Autodesk Inventor part; units mm, degrees
ref_plane "YZ Plane" through (0, 0, 0) normal (1, 0, 0) x (0, 1, 0)
ref_plane "XZ Plane" through (0, 0, 0) normal (0, 1, 0) x (-1, 0, 0)
ref_plane "XY Plane" through (0, 0, 0) normal (0, 0, 1) x (1, 0, 0)
sketch "Sketch1" plane through (0, 0, 0) normal (0, 1, 0) x (-1, 0, 0)
  line L0 (0, 0) -> (39, 0)
  line L1 (39, 0) -> (39, -51.8)
  line L2 (39, -51.8) -> (0, -51.8)
  line L3 (0, -51.8) -> (0, 0)
  dimension "d0" = 39
  dimension "d1" = 51.8
extrude "Extrusion1" add sketch "Sketch1" along normal blind 3
sketch "Sketch2" plane through (-39, 0, 0) normal (0, 0, 1) x (1, 0, 0)
  line L0 (0, 0) -> (30, 0)
  line L1 (30, 0) -> (30, 25)
  line L2 (30, 25) -> (0, 25)
  line L3 (0, 25) -> (0, 0)
  point P0 (39, 0)
  dimension "d4" = 25
extrude "Extrusion2" add sketch "Sketch2" along normal blind 3
sketch "Sketch3" plane through (-39, 0, 3) normal (0, 0, 1) x (1, 0, 0)
  line L0 (11.25, 19.8) -> (27.75, 19.8)
  line L1 (27.75, 19.8) -> (27.75, 5.8)
  line L2 (27.75, 5.8) -> (11.25, 5.8)
  line L3 (11.25, 5.8) -> (11.25, 19.8)
  line L4 (0, 0) -> (39, 0)
  line L5 (30, 0) -> (30, 25)
  dimension "d7" = 16.5
  dimension "d8" = 14
  dimension "d9" = 5.8
  dimension "d10" = 2.25
extrude "Extrusion3" cut sketch "Sketch3" against normal blind 3
sketch "Sketch5" plane through (-9, 3, 0) normal (1, 0, 0) x (0, 0, -1)
  line L0 (-3, -3) -> (-3, 22)
  line L1 (0, 0) -> (0, 22)
  line L2 (-3, -3) -> (0, -3)
  line L3 (0, -3) -> (0, 22)
  line L4 (0, 22) -> (-3, 22)
  line L5 (-3, 22) -> (-3, -3)
  point P0 (0, -3)
extrude "Extrusion4" add sketch "Sketch5" along normal blind 12
sketch "Sketch6" plane through (-39, 0, 3) normal (0, 0, 1) x (1, 0, 0)
  circle A0 centre (5, 12.5) radius 2
  circle A1 centre (37, 12.5) radius 2
  line L0 (0, 25) -> (0, 0)
  line L1 (42, 25) -> (42, 0)
  line L2 (0, 25) -> (42, 25)
  point P0 (39, 0)
  dimension "d15" = 4
  dimension "d16" = 4
  dimension "d17" = 5
  dimension "d18" = 5
  dimension "d19" = 12.5
  dimension "d20" = 12.5
extrude "Extrusion5" cut sketch "Sketch6" against normal blind 9
sketch "Sketch7" plane through (-39, 0, -51.8) normal (-1, 0, 0) x (0, 0, 1)
  line L0 (0, 0) -> (0, 3)
  line L1 (0, 3) -> (51.8, 3)
  line L2 (51.8, 3) -> (51.8, 0)
  line L3 (51.8, 0) -> (0, 0)
  line L4 (0, 0) -> (0, 3)
extrude "Extrusion6" add sketch "Sketch7" along normal blind 10
sketch "Sketch8" plane through (0, 3, 0) normal (0, 1, 0) x (1, 0, 0)
  circle A0 centre (-3, 31.478) radius 1.45
  circle A1 centre (-3, 6) radius 1.45
  circle A2 centre (-46, 31.4782) radius 1.45
  circle A3 centre (-46, 6) radius 1.45
  line L0 (0, 0) -> (0, 51.8)
  line L1 (-49, 0) -> (-49, 51.8)
  line L2 (-39, 0) -> (0, 0)
  line L3 (-39, 0) -> (-49, 0)
  dimension "d25" = 2.9
  dimension "d26" = 2.9
  dimension "d27" = 2.9
  dimension "d28" = 2.9
  dimension "d29" = 3
  dimension "d30" = 3
  dimension "d31" = 3
  dimension "d32" = 3
  dimension "d38" = 6
  dimension "d39" = 25.4782
  dimension "d40" = 25.478
  dimension "d41" = 6
extrude "Extrusion7" cut sketch "Sketch8" against normal blind 10
sketch "Sketch10" plane through (0, 0, -51.8) normal (0, 0, -1) x (-1, 0, 0)
  line L0 (-3, 25) -> (-3, 0)
  line L1 (0, 0) -> (49, 0)
  line L2 (49, 0) -> (49, 10)
  line L3 (49, 10) -> (0, 10)
  line L4 (0, 10) -> (0, 0)
  dimension "d35" = 10
extrude "Extrusion8" add sketch "Sketch10" along normal blind 3
sketch "Sketch11" plane through (-39, 0, 3) normal (-1, 0, 0) x (0, 0, 1)
  line L0 (0, 0) -> (-3, 0)
  line L1 (0, 0) -> (-3, 0)
  line L2 (-3, 0) -> (-3, 25)
  line L3 (-3, 25) -> (0, 25)
  line L4 (0, 25) -> (0, 0)
extrude "Extrusion9" add sketch "Sketch11" along normal blind 10
sketch "Sketch12" plane through (0, 0, 0) normal (1, 0, 0) x (0, 0, -1)
  line L0 (0, 3) -> (51.8, 3)
  line L1 (54.8, 0) -> (0, 0)
  line L2 (0, 0) -> (0, 3)
  line L3 (0, 3) -> (54.8, 3)
  line L4 (54.8, 3) -> (54.8, 0)
  point P0 (0, 0)
extrude "Extrusion10" add sketch "Sketch12" along normal blind 3
properties part number "SoporteEthernet"
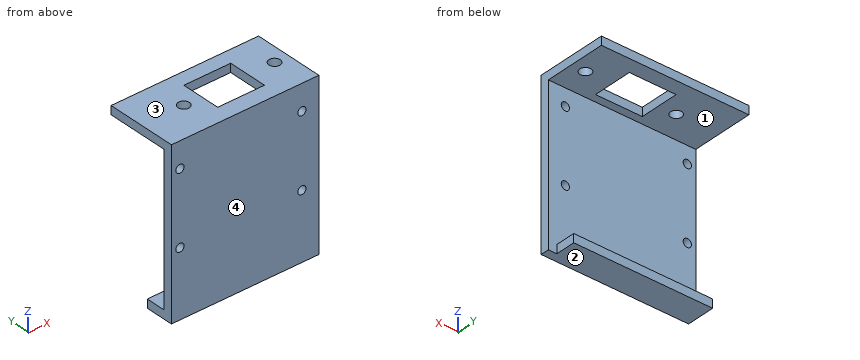
For this review, take the finished solid that the model builds, in its own axes (mm). Face numbers are marked on the shaded views. Round coordinates to 2 decimals unless told otherwise and drop trailing zeros. Loops run counter-clockwise (first coordinate to the right, second up) from the corner with the lowest first, then second, coordinate; pieces in that order, holes last. Notation, with made-up numbers: (-34, 57.25) - (-1, 57.25) arc R26 cw to (-1, 76.25) - close; hole circle Ø2 at (88, 12). An arc over 180 degrees is marked (long way). Use one line per item in the form item = value.
1) We need section B-B on y = 12.5. Write out the cut boundary in (x, z), then the cut area to 3 significant figures.
Solutions:
outline = (-49, 0) - (-36, 0) - (-36, 3) - (-49, 3) - close; (-32, 0) - (-27.75, 0) - (-27.75, 3) - (-32, 3) - close; (-11.25, 0) - (-4, 0) - (-4, 3) - (-11.25, 3) - close; (0, 0) - (3, 0) - (3, 3) - (0, 3) - close
area = 82.5 mm2
2) We need section A-A on x = -34. Write out the cut boundary in (y, z).
Solutions:
outline = (0, -54.8) - (10, -54.8) - (10, -51.8) - (3, -51.8) - (3, 0) - (10.5, 0) - (10.5, 3) - (0, 3) - close; (14.5, 0) - (25, 0) - (25, 3) - (14.5, 3) - close
3) Clearance check with flat-ended pins moving along their axes: P1, Ø3.5, axis at y = 7.5, z = -52.5, coming from the +X side; P2, Ø5, axis at x = -34, y = 12.5, coming from the +Z side; P3, Ø3.5, axis at x = -21, z = -54, coming from the +Y side; P4, Ø3.5, axis at x = -3, z = -31.478, coming from the +Y side. State where each tip first meets the part, or that it passes through.
Solutions:
P1 = 0
P2 = 3
P3 = 10
P4 = 3
4) Wall thickness on probe 1 along X at (y, z) = (0.7, -6); probe 2 along Z at (x, y) = (-36, 8); probe 3 along Y at (x, z) = (-34, 1.3): over which ranges is each line inside the solid? List them lowest first.
Solutions:
probe_1 = -49 to -47.45, -44.55 to -4.45, -1.55 to 3
probe_2 = -54.8 to -51.8, 0 to 3
probe_3 = 0 to 10.5, 14.5 to 25
5) We need section D-D on y = 18.75. Write out the cut boundary in (x, z).
Solutions:
outline = (-49, 0) - (-27.75, 0) - (-27.75, 3) - (-49, 3) - close; (-11.25, 0) - (3, 0) - (3, 3) - (-11.25, 3) - close
6) We need section C-C on x = -2.5. Write out the cut boundary in (y, z).
Solutions:
outline = (0, -54.8) - (10, -54.8) - (10, -51.8) - (3, -51.8) - (3, -32.84) - (0, -32.84) - close; (0, -30.12) - (3, -30.12) - (3, -7.36) - (0, -7.36) - close; (0, -4.64) - (3, -4.64) - (3, 0) - (10.56, 0) - (10.56, 3) - (0, 3) - close; (14.44, 0) - (25, 0) - (25, 3) - (14.44, 3) - close
7) Mouldability with a two-part tool opening along Z and no side actions: class the marked faces 1, 2, 3 and 4 as pulls with the +Z half, pulls with the -Z half, needs draft (parallel to the pull), parting line crosses it, or undercut.
Solutions:
face_1 = undercut
face_2 = pulls with the -Z half
face_3 = pulls with the +Z half
face_4 = needs draft
